Source: CAD feature listing. Evaluate the final solid. Frame: model axes, mm. Face numbers are marked on the shaded views. A direction names the side the tool comes from. Give positions to 0.01 mm unless a question says otherwise; leave off trailing zeros. Loops run counter-clockwise (first coordinate to the right, second up) from the corner with the lowest first, then second, coordinate; pieces in that order, holes last. Notation, with made-up numbers: M -23,-28 L 6,-28 A13 ccw 6,-19 Z; hole C 71,-0.75 d8. An arc over 180 degrees is marked long. Answer in a Markdown table with one row per item.
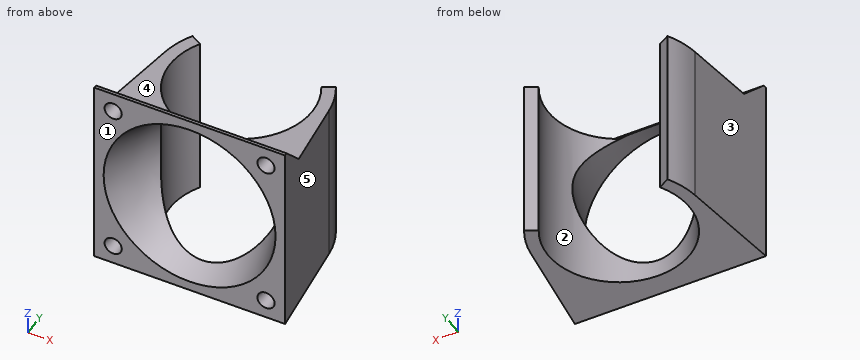
```python
from build123d import *

# Parameters (mm, degrees)
EXTRUDE_1_DEPTH               = 30
CUT_EXTRUDE_1_DEPTH           = 25
SKETCH_4_R                    = 1.35
CUT_EXTRUDE_3_DEPTH           = 8
CUT_EXTRUDE_3_DRAFT           = -8
CUT_EXTRUDE_3_PROFILE_2_DEPTH = 8
CUT_EXTRUDE_3_PROFILE_2_DRAFT = -8
CUT_EXTRUDE_3_PROFILE_3_DEPTH = 8
CUT_EXTRUDE_3_PROFILE_3_DRAFT = -8
CUT_EXTRUDE_3_PROFILE_4_DEPTH = 8
CUT_EXTRUDE_3_PROFILE_4_DRAFT = -8


with BuildPart() as part:
    # 草图1 → 凸台-拉伸1 (new body)
    with BuildSketch(Plane.XY):
        with BuildLine():
            Line((-9.526279442, 5.5), (-11.258330249, 6.5))
            ThreePointArc((-11.258330249, 6.5), (-12.31277123, 4.170811027), (-12.890950792, 1.680293923))
            Line((-12.890950792, 1.680293923), (-15, -14.5))
            Line((-15, -14.5), (15, -14.5))
            Line((15, -14.5), (12.890950792, 1.680293923))
            ThreePointArc((12.890950792, 1.680293923), (12.31277123, 4.170811027), (11.258330249, 6.5))
            Line((11.258330249, 6.5), (9.526279442, 5.5))
            ThreePointArc((9.526279442, 5.5), (0, -11), (-9.526279442, 5.5))
        make_face()
    extrude(amount=EXTRUDE_1_DEPTH)

    # 草图2 → 切除-拉伸1 (cut, symmetric)
    with BuildSketch(Plane(origin=(0, 0, 0), x_dir=(0, 0, -1), z_dir=(1, 0, 0))):
        Polygon((-30, -14), (-25.5, -9.5), (-25.5, 7.359440669), (-30, 7.359440669), align=None)
    extrude(amount=CUT_EXTRUDE_1_DEPTH, both=True, mode=Mode.SUBTRACT)

    # 切除-拉伸2 cone 1 section (through the dimple's axis) → 切除-拉伸2 (revolve, cut)
    with BuildSketch(Plane(origin=(0, -14.5, 15), x_dir=(0, 0, -1), z_dir=(1, 0, 0))):
        Polygon((0, 0), (13.5, 0), (0, 37.090945163), align=None)
    revolve(axis=Axis((0, -14.5, 15), (0, 1, 0)), mode=Mode.SUBTRACT)


with BuildPart() as cut_extrude_3_tool:
    # 草图4 → 切除-拉伸3 (with draft: the straight prism first)
    with BuildSketch(Plane.XZ.offset(14.5)):
        with Locations((-12, 27)):
            Circle(SKETCH_4_R)
    extrude(amount=-CUT_EXTRUDE_3_DEPTH)
    # 切除-拉伸3: the draft: its side faces are tilted about the plane it starts from
    cut_extrude_3_sides = [cut_extrude_3_tool.faces().sort_by_distance(p)[0] for p in [
        (-13.35, -10.5, 27),
    ]]
    draft(cut_extrude_3_sides, Plane.XZ.offset(14.5), CUT_EXTRUDE_3_DRAFT)


with BuildPart() as part_1:
    add(part.part)

    # 切除-拉伸3: cut by cut_extrude_3_tool
    add(cut_extrude_3_tool.part, mode=Mode.SUBTRACT)


with BuildPart() as cut_extrude_3_profile_2_tool:
    # 草图4 → 切除-拉伸3 profile 2 (with draft: the straight prism first)
    with BuildSketch(Plane.XZ.offset(14.5)):
        with Locations((12, 27)):
            Circle(SKETCH_4_R)
    extrude(amount=-CUT_EXTRUDE_3_PROFILE_2_DEPTH)
    # 切除-拉伸3 profile 2: the draft: its side faces are tilted about the plane it starts from
    cut_extrude_3_profile_2_sides = [cut_extrude_3_profile_2_tool.faces().sort_by_distance(p)[0] for p in [
        (10.65, -10.5, 27),
    ]]
    draft(cut_extrude_3_profile_2_sides, Plane.XZ.offset(14.5), CUT_EXTRUDE_3_PROFILE_2_DRAFT)


with BuildPart() as part_2:
    add(part_1.part)

    # 切除-拉伸3 profile 2: cut by cut_extrude_3_profile_2_tool
    add(cut_extrude_3_profile_2_tool.part, mode=Mode.SUBTRACT)


with BuildPart() as cut_extrude_3_profile_3_tool:
    # 草图4 → 切除-拉伸3 profile 3 (with draft: the straight prism first)
    with BuildSketch(Plane.XZ.offset(14.5)):
        with Locations((-12, 3)):
            Circle(SKETCH_4_R)
    extrude(amount=-CUT_EXTRUDE_3_PROFILE_3_DEPTH)
    # 切除-拉伸3 profile 3: the draft: its side faces are tilted about the plane it starts from
    cut_extrude_3_profile_3_sides = [cut_extrude_3_profile_3_tool.faces().sort_by_distance(p)[0] for p in [
        (-13.35, -10.5, 3),
    ]]
    draft(cut_extrude_3_profile_3_sides, Plane.XZ.offset(14.5), CUT_EXTRUDE_3_PROFILE_3_DRAFT)


with BuildPart() as part_3:
    add(part_2.part)

    # 切除-拉伸3 profile 3: cut by cut_extrude_3_profile_3_tool
    add(cut_extrude_3_profile_3_tool.part, mode=Mode.SUBTRACT)


with BuildPart() as cut_extrude_3_profile_4_tool:
    # 草图4 → 切除-拉伸3 profile 4 (with draft: the straight prism first)
    with BuildSketch(Plane.XZ.offset(14.5)):
        with Locations((12, 3)):
            Circle(SKETCH_4_R)
    extrude(amount=-CUT_EXTRUDE_3_PROFILE_4_DEPTH)
    # 切除-拉伸3 profile 4: the draft: its side faces are tilted about the plane it starts from
    cut_extrude_3_profile_4_sides = [cut_extrude_3_profile_4_tool.faces().sort_by_distance(p)[0] for p in [
        (10.65, -10.5, 3),
    ]]
    draft(cut_extrude_3_profile_4_sides, Plane.XZ.offset(14.5), CUT_EXTRUDE_3_PROFILE_4_DRAFT)


with BuildPart() as part_4:
    add(part_3.part)

    # 切除-拉伸3 profile 4: cut by cut_extrude_3_profile_4_tool
    add(cut_extrude_3_profile_4_tool.part, mode=Mode.SUBTRACT)


solid = part_4.part
```
1) Section C-C, the plane y = -8.25. Return loops of the section in (x, z), then the cut area to 3 significant figures.
Reply:
| item | result |
|---|---|
| outline | M -14.19,0 L -7.28,0 L -7.28,6.45 A11.23 cw -7.28,23.55 L -7.28,25.5 L -14.19,25.5 Z; M 7.28,0 L 14.19,0 L 14.19,25.5 L 7.28,25.5 L 7.28,23.55 A11.23 cw 7.28,6.45 Z; hole C -12,3 d0.94; hole C 12,3 d0.94 |
| area | 257 mm² |
2) Section D-D, the plane y = -12.5. Return loops of the section in (x, z), then the cut area to 3 significant figures.
Reply:
| item | result |
|---|---|
| outline | M -14.74,0 L 14.74,0 L 14.74,28.5 L -14.74,28.5 Z; hole C -12,3 d2.14; hole C -12,27 d2.14; hole C 0,15 d25.54; hole C 12,3 d2.14; hole C 12,27 d2.14 |
| area | 313 mm² |
3) Pull-direction query (X, two-part tool) for the marked faces 1, 2 and 3; classes: released by +X, released by -X, zero draft, split by the parting line, or undercut.
Reply:
| item | result |
|---|---|
| face 1 | zero draft |
| face 2 | undercut |
| face 3 | released by -X |
4) Set-up query: the marked faces 4 and 5. Return all of +Z, -Z, +X, -X, +Y, -Y with unobstructed straight access to the full face (end or side cutting, diameter ignored); none if empty.
Reply:
| item | result |
|---|---|
| face 4 | +Z, +X, -X, +Y |
| face 5 | +Z, -Z, +X, +Y |
5) Material intervals for L1, parallel to Z at x = 10.75, y = 3.5; L2, parallel to X at y = -7.5, z = 15; L3, parallel to Z at x = -9.75, y = -12.75, sorted ascending.
Reply:
| item | result |
|---|---|
| L1 | z = 0 to 25.5 |
| L2 | x = -14.09 to -10.95, 10.95 to 14.09 |
| L3 | z = 0 to 6.61, 23.39 to 28.75 |
6) Section B-B, the plane z = 15. Return loops of the section in (x, y).
Reply:
| item | result |
|---|---|
| outline | M -15,-14.5 L -13.5,-14.5 L -9.94,-4.71 A11 cw -9.53,5.5 L -11.26,6.5 A13 ccw -12.89,1.68 Z; M 9.53,5.5 A11 cw 9.94,-4.71 L 13.5,-14.5 L 15,-14.5 L 12.89,1.68 A13 ccw 11.26,6.5 Z |
7) Pin query (flat end, axial travel): pin 1 Ø2.5 at (x, y) = (-9.5, -4.5) entering from +Z; pin 2 Ø8 at (y, z) = (-8.5, 3.5) entering from -X; pin 3 Ø12 at (y, z) = (-12.5, 11) entering from +X; pin 4 Ø4 at (y, z) = (3, 6.5) entering from -X. Return the tip coordinate at first contact, or that it passes through.
Reply:
| item | result |
|---|---|
| pin 1 | stops at z = 25.5 |
| pin 2 | stops at x = -14.74 |
| pin 3 | stops at x = 15 |
| pin 4 | stops at x = -12.98 |
8) Section A-A, the plane y = -2.25. Return loops of the section in (x, z).
Reply:
| item | result |
|---|---|
| outline | M -13.4,0 L -10.77,0 L -10.77,25.5 L -13.4,25.5 Z; M 10.77,0 L 13.4,0 L 13.4,25.5 L 10.77,25.5 Z |
